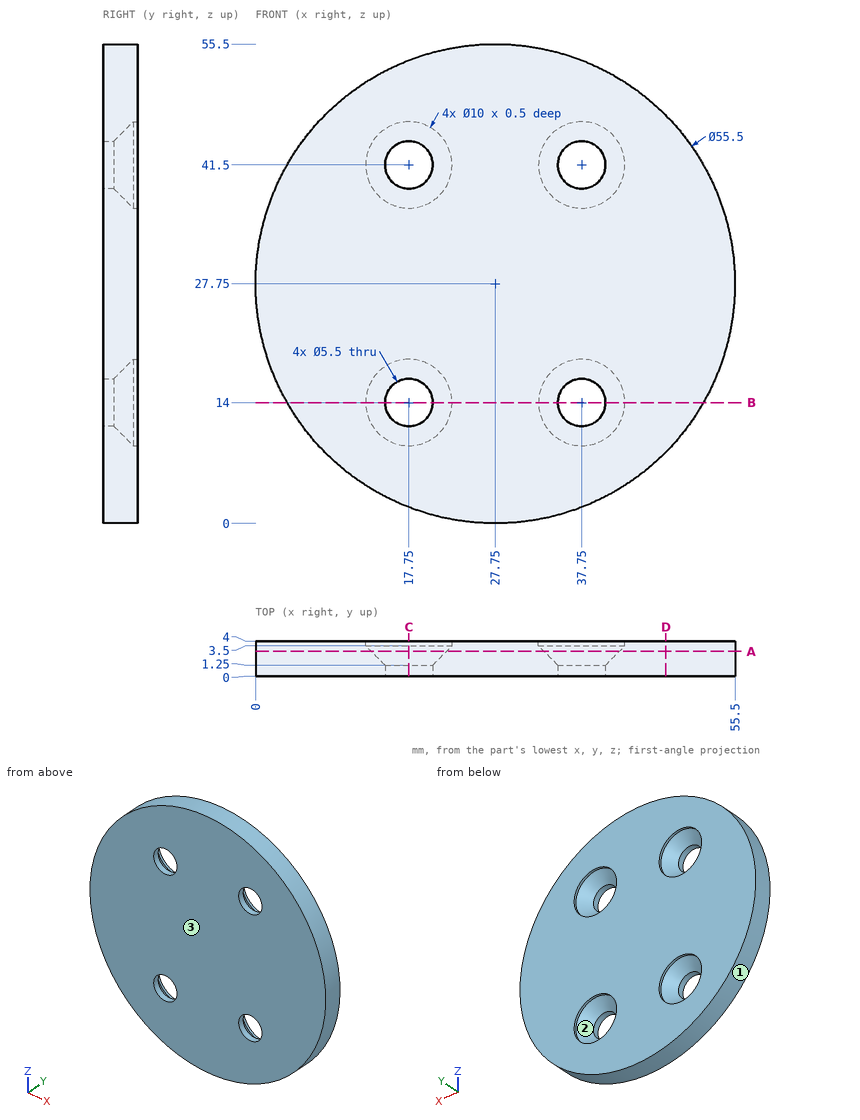
Part print with two shaded views. Sizes in mm from the minimum x, y, z corner. Coordinates: 2 decimals unless noted, no trailing zeros. Write each loop counter-clockwise with the first axis right and the second up, starting at its lowest first coordinate (ties: lowest second). Pieces come first, ordered by that corner, then holes.
1. Drop flat-ended pins along their axis: pin 1 (13 mm diameter, centred on x = 37.75, z = 14, fed in from -Y); pin 2 (2 mm diameter, centred on x = 41.5, y = 1.5, fed in from -Z); pin 3 (5 mm diameter, centred on x = 38.5, z = 43, fed in from +Y); pin 4 (2 mm diameter, centred on y = 2.5, z = 41.5, fed in from -X). Give the stop position or say it passes through.
Answer block:
pin 1: stops at y = 0
pin 2: stops at z = 3.1
pin 3: stops at y = 2.68
pin 4: stops at x = 3.1
2. Pull direction Z, two halves, no side cores. Call the marked faces 1, 2 and 3: released by +Z, released by -Z, zero draft, split by the parting line, or undercut.
Answer block:
face 1: split by the parting line
face 2: undercut
face 3: zero draft
3. Band-saw the part on D-D, the plane x = 47.5. Give the cut face in (y, z), and give its area (3 significant figures).
Answer block:
outline: (0, 8.26) - (4, 8.26) - (4, 47.24) - (0, 47.24) - close
area: 156 mm2
4. Drill centre lines: probe 1 along Z at (x, y) = (17.75, 0.5); probe 2 along Z at (x, y) = (20, 2.1); probe 3 along X at (y, z) = (2, 43). Where is each one in solid material? Low to high.
Answer block:
probe 1: z = 1.86 to 11.25, 16.75 to 38.75, 44.25 to 53.64
probe 2: z = 1.1 to 11.19, 16.81 to 38.69, 44.31 to 54.4
probe 3: x = 4.57 to 14.59, 20.91 to 34.59, 40.91 to 50.93
5. Band-saw the part on C-C, the plane x = 17.75. Give the cut face in (y, z), and give its area (3 significant figures).
Answer block:
outline: (0, 1.86) - (4, 1.86) - (4, 9) - (3.5, 9) - (1.25, 11.25) - (0, 11.25) - close; (0, 16.75) - (1.25, 16.75) - (3.5, 19) - (4, 19) - (4, 36.5) - (3.5, 36.5) - (1.25, 38.75) - (0, 38.75) - close; (0, 44.25) - (1.25, 44.25) - (3.5, 46.5) - (4, 46.5) - (4, 53.64) - (0, 53.64) - close
area: 148 mm2
6. Band-saw the part on A-A, the plane y = 2.85. Give the cut face in (x, z).
Answer block:
outline: circle Ø55.5 at (27.75, 27.75); hole circle Ø8.7 at (17.75, 14); hole circle Ø8.7 at (17.75, 41.5); hole circle Ø8.7 at (37.75, 14); hole circle Ø8.7 at (37.75, 41.5)
7. Band-saw the part on B-B, the plane z = 14. Give the cut face in (x, y), and give its area (3 significant figures).
Answer block:
outline: (3.65, 0) - (15, 0) - (15, 1.25) - (12.75, 3.5) - (12.75, 4) - (3.65, 4) - close; (20.5, 0) - (35, 0) - (35, 1.25) - (32.75, 3.5) - (32.75, 4) - (22.75, 4) - (22.75, 3.5) - (20.5, 1.25) - close; (40.5, 0) - (51.85, 0) - (51.85, 4) - (42.75, 4) - (42.75, 3.5) - (40.5, 1.25) - close
area: 134 mm2
